Check sheet for the modelled part. Datum: model origin and axes. Units: mm. A direction names the side the tool comes from. Round coordinates to 2 decimals unless told otherwise and drop trailing zeros. Order: outer loops, then holes, each group sorted by start corner. A loop starts at its lowest first (then second) coordinate and runs counter-clockwise, first axis right, second up. Notation, with made-up numbers: M 26,68 L 31,68 A21 cw 31,89 Z; hole C -3.75,-12 d3. An arc over 180 degrees is marked long. One line per item, written item: value. Start each with the question number.
(1) Cross-section at B-B, the plane y = -10. Enter the section's corners in (x, z), and give its area (3 significant figures).
(2) Thickness scan on L1, parallel to Y at x = 38.5, z = 44; L2, parallel to X at y = 7, z = 136; L3, parallel to X at y = -4.5, z = 134. Record the ranges inside material, lowest first.
(3) Cross-section at C-C, the plane x = 59.5. Enter the section's corners in (y, z).
(4) Depth check by flat-ended pin: pin 1 Ø12 at (y, z) = (-8, 84.5) entering from +X; pin 2 Ø8 at (y, z) = (10.5, 48) entering from -X; pin 3 Ø1.5 at (x, z) = (34, 104.5) entering from +Y; pin 4 Ø3 at (x, z) = (40.5, 86) entering from -Y. Enter the tip coordinate at first touch or a pass-through.
(5) Access from +Z, -Z, +X, -X, +Y, -Y to the whole of each face (thin tool, end or side, straight path). Record for faces 4 (the face through (40, 1, 74)), 5 (the face through (35.5, 6, 74)), 6 (the face through (34, 8, 74)).
(6) Release check for a two-part mould opening along Y. For faces 1 (the face through (44, 6, 150)), 2 (the face through (40, -1, 74)), 3 (the face through (38, -3, 74)) record: released by +Y, released by -Y, zero draft, split by the parting line, or undercut.
(7) Cross-section at A-A, the plane z = 24.5. Enter the section's corners in (x, y).
from build123d import *

# Parameters (mm, degrees)
PAD005_DEPTH            = 150
SKETCH013_R             = 14
POCKET005_DEPTH         = 150.001
SKETCH028_W             = 2
SKETCH028_H             = 10
POCKET010_DEPTH         = 150.001
BODY002_PLACEMENT_ANGLE = 90


with BuildPart() as part:
    # Sketch012 → Pad005 (new body)
    with BuildSketch(Plane.XY):
        with BuildLine():
            Line((-3, -3), (-8, -3))
            Line((-8, -3), (-8, 0))
            Line((-8, 0), (8, 0))
            Line((8, 0), (8, -3))
            Line((8, -3), (3, -3))
            Line((3, -3), (3, -8))
            ThreePointArc((-3, -8), (0, -41.733201), (3, -8))
            Line((-3, -3), (-3, -8))
        make_face()
    extrude(amount=PAD005_DEPTH)

    # Sketch013 (on Face10 of Pad005) → Pocket005 (cut, through all)
    with BuildSketch(Plane.XY.offset(150)):
        with Locations((0, -24.733201)):
            Circle(SKETCH013_R)
    extrude(amount=-POCKET005_DEPTH, mode=Mode.SUBTRACT)

    # Sketch028 (on Face4 of Pocket005) → Pocket010 (cut, through all)
    with BuildSketch(Plane(origin=(0, 0, 0), x_dir=(1, 0, 0), z_dir=(0, 0, -1))):
        with Locations((0, 10.103582)):
            Rectangle(SKETCH028_W, SKETCH028_H)
    extrude(amount=-POCKET010_DEPTH, mode=Mode.SUBTRACT)


with BuildPart() as part_1:
    # Body002 placement: moved
    add(part.part.moved(Location((32.5, 0, 0))).rotate(Axis((32.5, 0, 0), (0, 0, 1)), BODY002_PLACEMENT_ANGLE))


solid = part_1.part
Values found:
1. outline: M 43.49,0 L 47.44,0 L 47.44,150 L 43.49,150 Z; M 67.03,0 L 70.98,0 L 70.98,150 L 67.03,150 Z
1. area: 1,180 mm^2
2. L1: -3 to -1, 1 to 3
2. L2: 32.5 to 35.5, 41.74 to 45.11, 69.36 to 72.73
2. L3: 32.5 to 35.5, 40.84 to 43.98, 70.49 to 73.63
3. outline: M -16.85,0 L -13.82,0 L -13.82,150 L -16.85,150 Z; M 13.82,0 L 16.85,0 L 16.85,150 L 13.82,150 Z
4. pin 1: x = 74.12
4. pin 2: x = 32.5
4. pin 3: y = 8
4. pin 4: y = -7.55
5. face 4: +Z, -Z
5. face 5: +Z, -Z, +Y
5. face 6: +Z, -Z, -X, +Y
6. face 1: zero draft
6. face 2: undercut
6. face 3: released by -Y
7. outline: M 32.5,-8 L 35.5,-8 L 35.5,-3 L 40.5,-3 A17 ccw long 40.5,3 L 35.5,3 L 35.5,8 L 32.5,8 Z; hole M 37.6,-1 L 43.27,-1 A14 ccw long 43.27,1 L 37.6,1 Z
